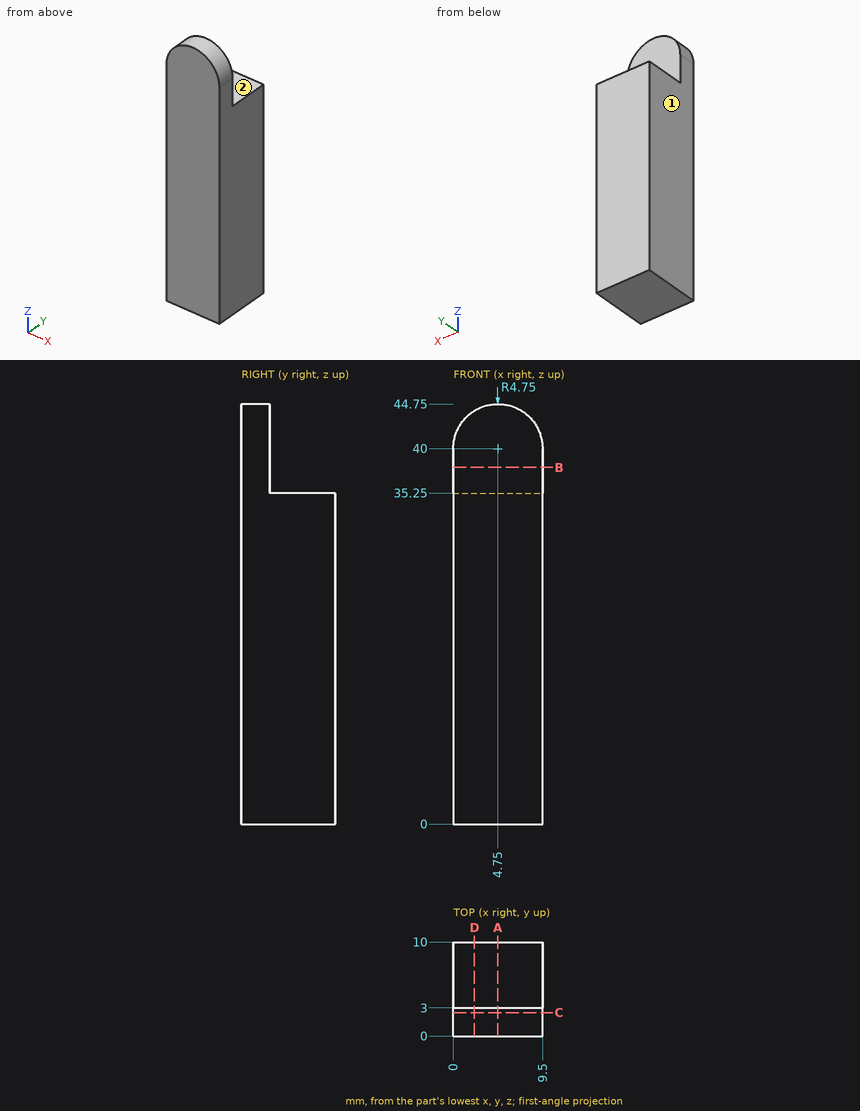
The figure shows three views and two pictorial views of one solid part (mm, origin at its lowest corner). Answer the questions. A direction names the side the tool comes from. Give positions to 0.01 mm unless a question says otherwise; leave off trailing zeros. Order: outer loops, then holes, each group sorted by start corner. A loop starts at its lowest first (then second) coordinate and runs counter-clockwise, first axis right, second up. Notation, with made-up numbers: (-0.75, 6) -> (51.25, 6) arc R16 cw to (51.25, 22) -> close; hole circle Ø9 at (-18.5, 88). An arc over 180 degrees is marked (long way). One line per item, written item: value.
1) Find section C-C, the plane y = 2.5. Determine the outline of the cut face in (x, z).
Reported:
outline: (0, 0) -> (9.5, 0) -> (9.5, 40) arc R4.75 ccw to (0, 40) -> close
2) Find section B-B, the plane z = 38. Determine the outline of the cut face in (x, y).
Reported:
outline: (0, 0) -> (9.5, 0) -> (9.5, 3) -> (0, 3) -> close
3) Find section A-A, the plane x = 4.75. Determine the outline of the cut face in (y, z), plus the area to 3 significant figures.
Reported:
outline: (0, 0) -> (10, 0) -> (10, 35.25) -> (3, 35.25) -> (3, 44.75) -> (0, 44.75) -> close
area: 381 mm^2
4) Find section D-D, the plane x = 2.25. Determine the outline of the cut face in (y, z), plus the area to 3 significant figures.
Reported:
outline: (0, 0) -> (10, 0) -> (10, 35.25) -> (3, 35.25) -> (3, 44.04) -> (0, 44.04) -> close
area: 379 mm^2
5) A tool of negligible diameter and unlimited length cuts with its end or side. For the marked faces 1 and 2, from which of +Z, -Z, +X, -X, +Y, -Y can it reach the whole face along a straight path? Write none if from no direction.
Reported:
face 1: +Z, -Z, -X, +Y, -Y
face 2: +Z, +X, -X, +Y
6) Flat-ended cylindrical pins translate along their axes: P1, Ø3, axis at y = 8, z = 38, coming from the -X side; P2, Ø3.5, axis at x = 5.5, y = 5, coming from the +Z side. Find the tip coordinate at first contact, or state that the pin passes through.
Reported:
P1: passes through
P2: stops at z = 35.25
7) Find the intervals of material crossed by line 1 (Z direction, x = 8, y = 4); line 2 (Y direction, x = 4, z = 37); line 3 (Z direction, x = 1, y = 2.5), in increasing order.
Reported:
line 1: z = 0 to 35.25
line 2: y = 0 to 3
line 3: z = 0 to 42.92
